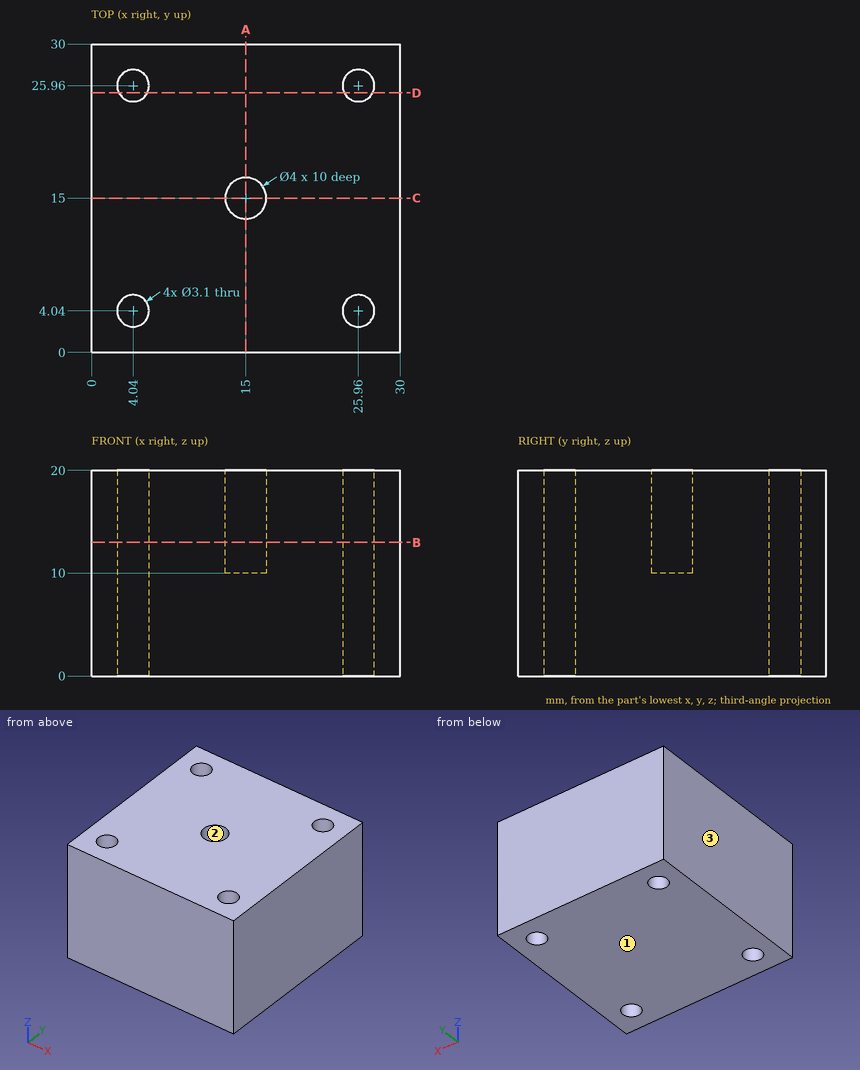
Answer from the drawing. Dimensions are ordinates in mm from the lowest x, y and z of the part. Coordinates: 2 decimals unless noted, no trailing zeros. Loops run counter-clockwise (first coordinate to the right, second up) from the corner with the lowest first, then second, coordinate; pieces in that order, holes last.
1) Section D-D (y = 25.25) is taken. Give the vertices of the cut face in (x, z).
Results:
outline: (0, 0) - (2.66, 0) - (2.66, 20) - (0, 20) - close; (5.42, 0) - (24.58, 0) - (24.58, 20) - (5.42, 20) - close; (27.34, 0) - (30, 0) - (30, 20) - (27.34, 20) - close
2) Consider probe 1 along X at (y, z) = (26.75, 14.5); probe 2 along Y at (x, z) = (15, 14.5); probe 3 along X at (y, z) = (26.5, 7.75). Determine where each line is inside the solid, lowest interval first.
Results:
probe 1: x = 0 to 2.71, 5.37 to 24.63, 27.29 to 30
probe 2: y = 0 to 13, 17 to 30
probe 3: x = 0 to 2.59, 5.49 to 24.51, 27.41 to 30
3) For a pull along X with two mould halves and no side action, classify the marked faces 1, 2 and 3 as +X half, -X half, draft (parallel to the pull), parting line (faces both ways), or undercut.
Results:
face 1: draft
face 2: undercut
face 3: -X half
4) Section A-A (x = 15) is taken. Give the vertices of the cut face in (y, z).
Results:
outline: (0, 0) - (30, 0) - (30, 20) - (17, 20) - (17, 10) - (13, 10) - (13, 20) - (0, 20) - close
5) A flat-ended cylindrical pin translates along its axis: pin 1 (3 mm diameter, centred on x = 15, y = 15, fed in from +Z). Find the tip coordinate at first contact, or state that the pin passes through.
Results:
pin 1: stops at z = 10
6) Section B-B (z = 13) is taken. Give the vertices of the cut face in (x, y), plus the area to 3 significant figures.
Results:
outline: (0, 0) - (30, 0) - (30, 30) - (0, 30) - close; hole circle Ø3.1 at (4.04, 4.04); hole circle Ø3.1 at (4.04, 25.96); hole circle Ø4 at (15, 15); hole circle Ø3.1 at (25.96, 4.04); hole circle Ø3.1 at (25.96, 25.96)
area: 857 mm2
